Geometry: final body of the model. Coordinates: model frame, mm. A direction names the side the tool comes from. Round coordinates to 2 decimals unless told otherwise and drop trailing zeros. Loops run counter-clockwise (first coordinate to the right, second up) from the corner with the lowest first, then second, coordinate; pieces in that order, holes last. Notation, with made-up numbers: M 55,49 L 86,49 A9 cw 86,55 Z; hole C 52,82 d5. An arc over 180 degrees is marked long. Answer as a JSON object with one key per item and string values.
```python
from build123d import *
from OCP.BRepFilletAPI import BRepFilletAPI_MakeChamfer

# Parameters (mm, degrees)
BOSS_EXTRUDE1_START  = 2
SKETCH1_W            = 17.5768
SKETCH1_H            = 31.241999999999997
SKETCH1_W_2          = 15.036799999999998
SKETCH1_H_2          = 24.764999999999997
BOSS_EXTRUDE1_DEPTH  = 2
BOSS_EXTRUDE2_START  = 2
BOSS_EXTRUDE2_DEPTH  = 29.09
BOSS_EXTRUDE3_DEPTH  = 1.5
BOSS_EXTRUDE4_DEPTH  = 13.843
BOSS_EXTRUDE5_DEPTH  = 1.095
BOSS_EXTRUDE6_DEPTH  = 1.095
BOSS_EXTRUDE7_DEPTH  = 2
CHAMFER1_SIZE        = 2.3
CHAMFER1_SIZE2       = 0.8
BOSS_EXTRUDE9_DEPTH  = 5.299999999999998
CHAMFER2_SIZE        = 1.8
CUT_EXTRUDE1_DEPTH   = 0.25
CUT_EXTRUDE2_DEPTH   = 0.25
CUT_EXTRUDE3_REACH   = 62.791
SKETCH15_W           = 2.073672467648368
SKETCH15_H           = 2.532
BOSS_EXTRUDE10_DEPTH = 2
CHAMFER3_SIZE        = 0.3
CHAMFER4_SIZE        = 2


with BuildPart() as part:
    # Sketch1 → Boss-Extrude1 (new body)
    with BuildSketch(Plane.XY.offset(BOSS_EXTRUDE1_START)):
        with Locations((12.544999999999998, 29.464000000000002)):
            Rectangle(SKETCH1_W, SKETCH1_H)
        with Locations((12.544999999999998, 31.051499999999997)):
            Rectangle(SKETCH1_W_2, SKETCH1_H_2, mode=Mode.SUBTRACT)
    extrude(amount=BOSS_EXTRUDE1_DEPTH)



with BuildPart() as body_2:
    # Sketch2 → Boss-Extrude2 (new body)
    with BuildSketch(Plane(origin=(25.09, 5.28e-15, 0), x_dir=(0, 0, -1), z_dir=(1, 2.1e-16, 0)).offset(BOSS_EXTRUDE2_START)):
        with BuildLine():
            Line((0, 51.489999999999995), (2.4e-16, 49.489999999999995))
            Line((2.4e-16, 49.489999999999995), (-4, 49.489999999999995))
            Line((-4, 49.489999999999995), (-4.000000000000001, 53.99431457505075))
            Line((-4.000000000000001, 53.99431457505075), (0.7579894972000346, 53.99431457505075))
            Line((0.7579894972000346, 53.99431457505075), (2.805084072136604, 51.947220000114164))
            Line((2.805084072136604, 51.947220000114164), (2.805084072136603, 51.02508407213661))
            Line((2.805084072136603, 51.02508407213661), (2.552842712474611, 50.77284271247461))
            ThreePointArc((2.552842712474611, 50.77284271247461), (2.2699999999999894, 50.65568542494923), (1.9871572875253678, 50.77284271247461))
            Line((1.9871572875253678, 50.77284271247461), (1.27, 51.489999999999995))
            Line((1.27, 51.489999999999995), (0.6828427124746198, 52.07715728752538))
            ThreePointArc((0.6828427124746198, 52.07715728752538), (0.24692662705396132, 52.163866388055276), (0, 51.794314575050755))
            Line((0, 51.794314575050755), (0, 51.489999999999995))
        make_face()
    extrude(amount=-BOSS_EXTRUDE2_DEPTH)


with BuildPart() as body_3:
    # Sketch4 → Boss-Extrude3 (new body)
    with BuildSketch(Plane.XZ):
        Polygon((6.374999999999999, 4), (18.715, 4), (18.715, -1.7), (6.374999999999999, -1.699999999999999), align=None)
        with BuildLine():
            Line((17.215, 1.2499999999999993), (17.214999999999996, 1.96))
            ThreePointArc((17.214999999999996, 1.96), (16.79030483272049, 2.985304832720491), (15.765, 3.409999999999999))
            Line((15.765, 3.409999999999999), (9.325, 3.41))
            ThreePointArc((9.325, 3.41), (8.299695167279506, 2.985304832720494), (7.875, 1.96))
            Line((7.875, 1.96), (7.874999999999998, 1.2499999999999998))
            ThreePointArc((7.874999999999998, 1.2499999999999998), (8.299695167279504, 0.22469516727950523), (9.325, -0.20000000000000095))
            Line((9.325, -0.20000000000000095), (15.765, -0.19999999999999923))
            ThreePointArc((15.765, -0.19999999999999923), (16.790304832720494, 0.22469516727950656), (17.215, 1.2499999999999993))
        make_face(mode=Mode.SUBTRACT)
    extrude(amount=BOSS_EXTRUDE3_DEPTH)


with BuildPart() as part_1:
    add(part.part)

    add(body_3.part)  # Boss-Extrude4 merges body 3
    # Sketch5 → Boss-Extrude4 (add)
    with BuildSketch(Plane(origin=(0, 0, 0), x_dir=(1, 1.4e-16, 0), z_dir=(-1.4e-16, 1, 0))):
        with BuildLine():
            ThreePointArc((9.325, -3.41), (8.31393620379325, -2.9993507588874895), (7.875551829143242, -2))
            Line((7.875551829143242, -2), (6.374999999999999, -2))
            Line((6.374999999999999, -2), (6.374999999999999, -4))
            Line((6.375, -4), (18.715, -4))
            Line((18.715, -4), (18.715, -2))
            Line((18.715, -2), (17.214448170856755, -2))
            ThreePointArc((17.214448170856755, -2), (16.77606379620675, -2.9993507588874895), (15.765, -3.4099999999999993))
            Line((15.765, -3.409999999999999), (9.325, -3.4099999999999997))
        make_face()
    extrude(amount=BOSS_EXTRUDE4_DEPTH)

    # Sketch6 → Boss-Extrude5 (add)
    with BuildSketch(Plane.XY.offset(2.905)):
        Polygon((6.1249999999999964, 13.843), (6.124999999999998, -1.4999999999999991), (1.821e-14, -1.5), (1.431e-14, 13.843), align=None)
    extrude(amount=BOSS_EXTRUDE5_DEPTH)

    # Sketch9 → Boss-Extrude6 (add)
    with BuildSketch(Plane.XY.offset(2.905)):
        Polygon((18.965, 13.843), (25.09, 13.843), (25.09, -1.4999999999999973), (18.965000000000003, -1.4999999999999973), align=None)
    extrude(amount=BOSS_EXTRUDE6_DEPTH)


    add(body_2.part)  # Boss-Extrude7 merges body 2
    # Sketch10 → Boss-Extrude7 (add)
    with BuildSketch(Plane.XY.offset(4)):
        Polygon((25.09, 49.489999999999995), (25.09, 13.843), (21.333399999999997, 13.843), (21.333399999999997, 45.085), (3.7566, 45.085), (3.7566, 13.843), (1.431e-14, 13.843), (-8.67e-15, 49.489999999999995), align=None)
    extrude(amount=-BOSS_EXTRUDE7_DEPTH)

    # Chamfer1: one chamfer whose edges measure the first distance from different faces: ONE call of the kernel's chamfer builder (chamfer() names one face for all edges)
    chamfer1_edges_1 = [part_1.edges().sort_by_distance(p)[0] for p in [
        (22.0275, 13.843, 2.905),
    ]]
    chamfer1_side_1 = [part_1.faces().sort_by_distance(p)[0] for p in [
        (22.0275, 6.171500000000002, 2.905),
    ]]
    chamfer1_edges_2 = [part_1.edges().sort_by_distance(p)[0] for p in [
        (3.0625000000000053, 13.843, 2.905),
    ]]
    chamfer1_side_2 = [part_1.faces().sort_by_distance(p)[0] for p in [
        (3.0625000000000067, 6.1715, 2.9050000000000002),
    ]]
    chamfer1 = BRepFilletAPI_MakeChamfer(part_1.part.solid().wrapped)
    for e in chamfer1_edges_1:
        chamfer1.Add(CHAMFER1_SIZE, CHAMFER1_SIZE2, e.wrapped, chamfer1_side_1[0].wrapped)  # the first distance lies on this face
    for e in chamfer1_edges_2:
        chamfer1.Add(CHAMFER1_SIZE, CHAMFER1_SIZE2, e.wrapped, chamfer1_side_2[0].wrapped)  # the first distance lies on this face
    add(Compound.cast(chamfer1.Shape()), mode=Mode.REPLACE)

    # Sketch11 → Boss-Extrude9 (add)
    with BuildSketch(Plane(origin=(0, 0, 2.905), x_dir=(-1, 0, 0), z_dir=(0, 0, -1))):
        Polygon((-6.124999999999998, -1.4999999999999991), (-1.779e-14, -1.4999999999999991), (-1.49e-14, 0.2500000000000002), (-6.124999999999998, 0.2500000000000009), align=None)
        Polygon((-18.965000000000003, -1.4999999999999973), (-25.09, -1.4999999999999973), (-25.09, 0.25000000000000194), (-18.965000000000003, 0.25000000000000266), align=None)
    extrude(amount=BOSS_EXTRUDE9_DEPTH)

    # Chamfer2
    chamfer2_edges = [part_1.edges().sort_by_distance(p)[0] for p in [
        (3.0625000000000067, 0.25000000000000056, 2.905),
        (22.027500000000003, 0.2500000000000023, 2.905),
    ]]
    chamfer(chamfer2_edges, length=CHAMFER2_SIZE)

    # Sketch12 → Cut-Extrude1 (cut)
    with BuildSketch(Plane(origin=(6.124999999999998, 6.9e-16, 0), x_dir=(0, 0, -1), z_dir=(1, 1.1e-16, 0))):
        Polygon((-4, 13.843), (-4, -1.4999999999999998), (2.3949999999999987, -1.4999999999999998), (2.3949999999999987, 0.25000000000000017), (-1.1049999999999898, 0.25000000000000017), (-2.905, 2.0499999999999883), (-2.905, 11.543000000000012), (-2.104999999999996, 13.843), align=None)
    extrude(amount=-CUT_EXTRUDE1_DEPTH, mode=Mode.SUBTRACT)

    # Sketch13 → Cut-Extrude2 (cut)
    with BuildSketch(Plane.ZY.offset(-18.965000000000003)):
        Polygon((4, -1.5000000000000018), (4, 13.842999999999996), (2.104999999999996, 13.842999999999996), (2.905, 11.543000000000008), (2.905, 2.04999999999999), (1.1049999999999898, 0.2499999999999984), (-2.3949999999999987, 0.2499999999999984), (-2.3949999999999987, -1.5000000000000018), align=None)
    extrude(amount=-CUT_EXTRUDE2_DEPTH, mode=Mode.SUBTRACT)

    # Cut-Extrude3: up to this face of the body (flat: up to its plane)
    cut_extrude3_end = Plane(part_1.part.faces().sort_by_distance((2.9375, -0.625, -2.395))[0])
    # Sketch14 → Cut-Extrude3 (cut, up to the picked face)
    with BuildSketch(Plane.XY.offset(3.9999999999999907), mode=Mode.PRIVATE) as cut_extrude3_sk1:
        Polygon((25.09, 18.669), (24.79, -1.4999999999999967), (25.09, -1.4999999999999967), align=None)
    cut_extrude3_tool1 = split(extrude(cut_extrude3_sk1.sketch, amount=-CUT_EXTRUDE3_REACH, mode=Mode.PRIVATE), bisect_by=cut_extrude3_end, keep=Keep.BOTH, mode=Mode.PRIVATE)
    # Sketch14 → Cut-Extrude3 (cut, up to the picked face)
    with BuildSketch(Plane.XY.offset(3.9999999999999907), mode=Mode.PRIVATE) as cut_extrude3_sk2:
        Polygon((-1.119e-14, 18.669755162923135), (0.3000000000000182, -1.4999999999999993), (1.821e-14, -1.4999999999999991), align=None)
    cut_extrude3_tool2 = split(extrude(cut_extrude3_sk2.sketch, amount=-CUT_EXTRUDE3_REACH, mode=Mode.PRIVATE), bisect_by=cut_extrude3_end, keep=Keep.BOTH, mode=Mode.PRIVATE)
    add(cut_extrude3_tool1.solids().sort_by(Axis((24.99, 5.223, 4), (0, 0, -1)))[0], mode=Mode.SUBTRACT)
    add(cut_extrude3_tool2.solids().sort_by(Axis((0.1, 5.223252, 4), (0, 0, -1)))[0], mode=Mode.SUBTRACT)

    # Sketch15 → Boss-Extrude10 (add)
    with BuildSketch(Plane.XY.offset(3.9999999999999907)):
        with Locations((26.00316376617581, 11.620500000000002)):
            Rectangle(SKETCH15_W, SKETCH15_H)
    extrude(amount=-BOSS_EXTRUDE10_DEPTH)

    # Chamfer3
    chamfer3_edges = [part_1.edges().sort_by_distance(p)[0] for p in [
        (6.374999999999998, 6.171500000000002, 4),
        (18.714999999999996, 6.171500000000003, 4),
    ]]
    chamfer(chamfer3_edges, length=CHAMFER3_SIZE)

    # Chamfer4
    chamfer4_edges = [part_1.edges().sort_by_distance(p)[0] for p in [
        (7.1252759145716205, 1e-15, 2),
        (17.96472408542838, 2.53e-15, 2),
    ]]
    chamfer(chamfer4_edges, length=CHAMFER4_SIZE)


solid = part_1.part
```
1) Line query: probe 1 along X at (y, z) = (22.5, 2.25); probe 2 along Y at (x, z) = (7, -0.5); probe 3 along Y at (x, z) = (17.25, 2.5). Output: solid intervals per line, ascending.
Geometry results:
{"probe 1": "0 to 5.03, 20.06 to 25.09", "probe 2": "-1.5 to 0, 52.18 to 53.99", "probe 3": "-1.5 to 18.67, 43.43 to 53.99"}
2) Pull-direction query (Y, two-part tool) for faces 5 (the face through (22.16, 12.71, 2.5)), 6 (the face through (6.375, 4.4, 2.2)), 7 (the face through (12, 13.843, 3)); classes: +Y half, -Y half, draft (parallel to the pull), parting line (faces both ways), or undercut.
Geometry results:
{"face 5": "undercut", "face 6": "draft", "face 7": "-Y half"}
3) Cut plane C-C on x = 14.75. Return the cut outline in (y, z).
Geometry results:
{"outline": "M -1.5,-1.7 L 0,-1.7 L 0,-0.2 L -1.5,-0.2 Z; M -1.5,3.41 L 13.84,3.41 L 13.84,2 L 18.67,2 L 18.67,4 L -1.5,4 Z; M 43.43,2 L 49.49,2 L 49.49,0 L 51.79,0 A0.4 cw 52.08,-0.68 L 50.77,-1.99 A0.4 ccw 50.77,-2.55 L 51.03,-2.81 L 51.95,-2.81 L 53.99,-0.76 L 53.99,4 L 43.43,4 Z"}
4) Cut plane D-D on x = 3.75. Return the cut outline in (y, z) (3 decimals), and give its area (3 significant figures).
Geometry results:
{"outline": "M -1.5,-2.395 L 0.25,-2.395 L 0.25,1.105 L 2.05,2.905 L 11.543,2.905 L 13.843,2.105 L 13.843,2 L 49.49,2 L 49.49,0 L 51.794,0 A0.4 cw 52.077,-0.683 L 50.773,-1.987 A0.4 ccw 50.773,-2.553 L 51.025,-2.805 L 51.947,-2.805 L 53.994,-0.758 L 53.994,4 L -1.5,4 Z", "area": "123 mm2"}
5) First-contact query: pin 1 (1.9 mm diameter, centred on x = 23, y = -0.5, fed in from -Z) (3 decimals); pin 2 (1.6 mm diameter, centred on x = 12.5, y = -0.5, fed in from -Z); pin 3 (0.7 mm diameter, centred on y = 12, z = 2.5, fed in from -X). Flat tips, straight axial feed; report the tip coordinate or a pass-through.
Geometry results:
{"pin 1": "z = -2.395", "pin 2": "z = -1.7", "pin 3": "x = 0.09"}
6) Cut plane B-B on x = 7.25. Return the cut outline in (y, z).
Geometry results:
{"outline": "M -1.5,-1.7 L 0,-1.7 L 0,0 L 2,2 L 18.67,2 L 18.67,4 L -1.5,4 Z; M 43.43,2 L 49.49,2 L 49.49,0 L 51.79,0 A0.4 cw 52.08,-0.68 L 50.77,-1.99 A0.4 ccw 50.77,-2.55 L 51.03,-2.81 L 51.95,-2.81 L 53.99,-0.76 L 53.99,4 L 43.43,4 Z"}
7) Cut plane A-A on y = 29. Return the cut outline in (x, z), and give its area (3 significant figures).
Geometry results:
{"outline": "M 0,2 L 5.03,2 L 5.03,4 L 0,4 Z; M 20.06,2 L 25.09,2 L 25.09,4 L 20.06,4 Z", "area": "20.1 mm2"}
8) Set-up query: faces 1 (the face through (13, -1, -1.7)), 2 (the face through (12, 18.669, 3)), 3 (the face through (19.215, 3.9, 3.2)), 4 (the face through (22, -1, -2.395)). Return all of +Z, -Z, +X, -X, +Y, -Y with unobstructed straight access to the full face (end or side cutting, diameter ignored); none if empty.
Geometry results:
{"face 1": "-Z, -Y", "face 2": "+Z, -Z", "face 3": "+Z, -Z, -Y", "face 4": "-Z, +X, -X, -Y"}
